Could you check a few things on this drawing? It's one solid part, dimensions in mm from its lowest x, y, z. Give positions to 0.01 mm unless a question says otherwise; leave off trailing zeros. Loops run counter-clockwise (first coordinate to the right, second up) from the corner with the lowest first, then second, coordinate; pieces in that order, holes last.
1. Imagine slicing it at D-D (z = 1.5). List the corners of the cut face in (x, y) for me, plus the area to 3 significant figures.
2. Imagine slicing it at A-A (z = 3.25). List the corners of the cut face in (x, y) for me.
3. For P1, Ø0.5, axis at x = 1.5, z = 9.5, coming from the +Y side; P2, Ø0.5, axis at y = 1, z = 8, coming from the +X side, each with a flat end and sliding along its axis, tell me the tip position at first contact or that it passes through.
4. I need wall thicknesses on line 1 along Z through (x, y) = (2.35, 1.2); line 2 along X through (y, z) = (1.15, 9.5). Which ranges of each line are inside material? Lowest first, please.
5. Imagine slicing it at B-B (x = 1.27). List the corners of the cut face in (y, z) for me, plus the area to 3 significant figures.
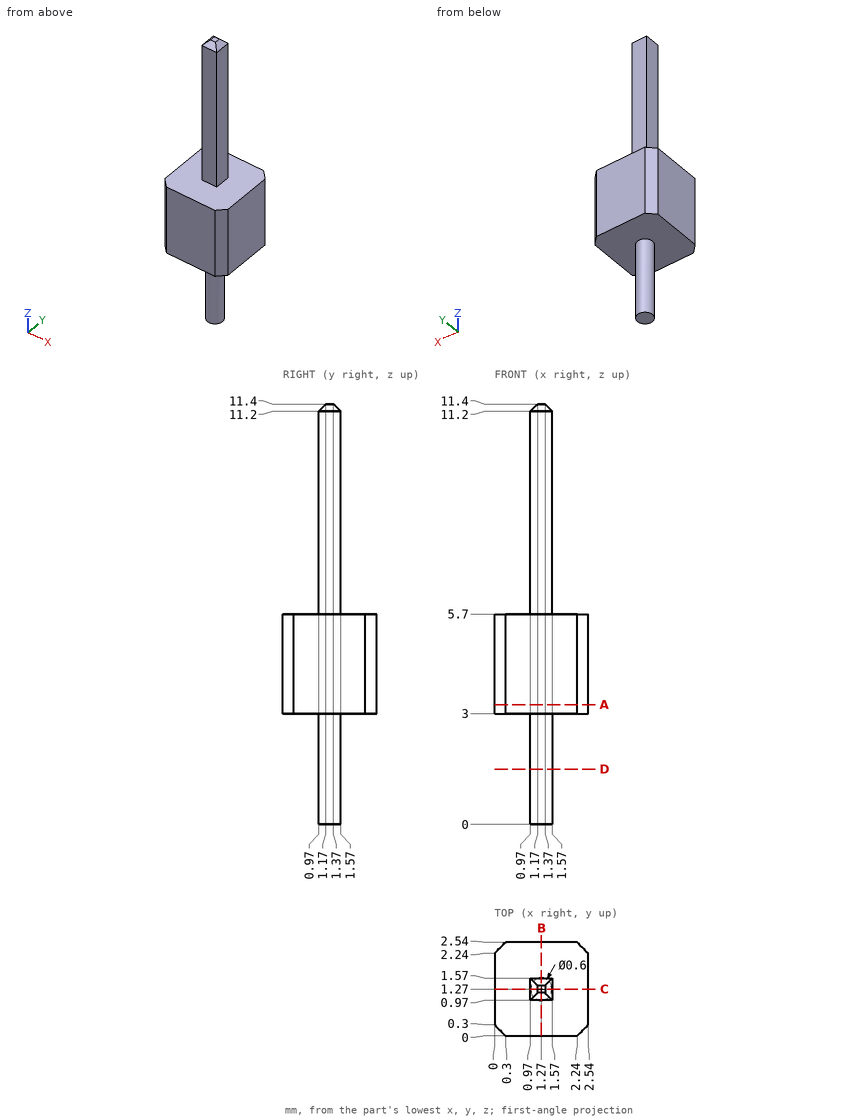
Derived:
1. outline: circle Ø0.6 at (1.27, 1.27)
1. area: 0.283 mm2
2. outline: (0, 0.3) - (0.3, 0) - (2.24, 0) - (2.54, 0.3) - (2.54, 2.24) - (2.24, 2.54) - (0.3, 2.54) - (0, 2.24) - close
3. P1: stops at y = 1.57
3. P2: stops at x = 1.57
4. line 1: z = 3 to 5.7
4. line 2: x = 0.97 to 1.57
5. outline: (0, 3) - (0.97, 3) - (0.97, 0) - (1.57, 0) - (1.57, 3) - (2.54, 3) - (2.54, 5.7) - (1.57, 5.7) - (1.57, 11.2) - (1.37, 11.4) - (1.17, 11.4) - (0.97, 11.2) - (0.97, 5.7) - (0, 5.7) - close
5. area: 12.0 mm2
